Verification items for the finished model (mm, model axes). Round coordinates to 2 decimals unless told otherwise and drop trailing zeros. Loops run counter-clockwise (first coordinate to the right, second up) from the corner with the lowest first, then second, coordinate; pieces in that order, holes last. Notation, with made-up numbers: (77.25, -26.75) -> (136.25, -26.75) arc R20 cw to (136.25, 2.25) -> close; hole circle Ø2 at (-3.5, 19.5). An arc over 180 degrees is marked (long way). Use a Markdown table: item, result. Add a question column.
```python
from build123d import *

# Parameters (mm, degrees)
F0_R     = 44.45
F0_R_2   = 1.5
F0_R_3   = 2.5
F1_DEPTH = 3.175


# Not quite as in the source:
# - a length typed as a fraction of an inch, garbled in the dataset ("3 / 203.2 mm" for 3/8 in), is restored


with BuildPart() as f1:
    # F0 (on Front) → F1 (new body)
    with BuildSketch(Plane.XZ):
        Circle(F0_R)
        with Locations((-19.725, -34.1647021793)):
            Circle(F0_R_2, mode=Mode.SUBTRACT)
        with Locations((-34.1647021793, -19.725)):
            Circle(F0_R_2, mode=Mode.SUBTRACT)
        with Locations((0, -39.45)):
            Circle(F0_R_2, mode=Mode.SUBTRACT)
        with Locations((19.725, -34.1647021793)):
            Circle(F0_R_2, mode=Mode.SUBTRACT)
        Polygon((10, -27.5), (10, -15), (10, -2.5), (13.175, -2.5), (13.175, -15), (13.175, -27.5), align=None, mode=Mode.SUBTRACT)
        with Locations((34.1647021793, -19.725)):
            Circle(F0_R_2, mode=Mode.SUBTRACT)
        with Locations((-39.45, 0)):
            Circle(F0_R_2, mode=Mode.SUBTRACT)
        with Locations((-24.125, 9.91)):
            Circle(F0_R_3, mode=Mode.SUBTRACT)
        with Locations((-34.1647021793, 19.725)):
            Circle(F0_R_2, mode=Mode.SUBTRACT)
        with Locations((-24.125, 19.91)):
            Circle(F0_R_3, mode=Mode.SUBTRACT)
        with Locations((-19.725, 34.1647021793)):
            Circle(F0_R_2, mode=Mode.SUBTRACT)
        Polygon((-20, 15.91), (-20, 24.82), (20, 24.82), (20, 15.91), (30, 15.91), (30, 13.91), (20, 13.91), (20, 5), (-20, 5), (-20, 13.91), (-30, 13.91), (-30, 15.91), align=None, mode=Mode.SUBTRACT)
        with Locations((24.125, 9.91)):
            Circle(F0_R_3, mode=Mode.SUBTRACT)
        with Locations((39.45, 0)):
            Circle(F0_R_2, mode=Mode.SUBTRACT)
        with Locations((24.125, 19.91)):
            Circle(F0_R_3, mode=Mode.SUBTRACT)
        with Locations((34.1647021793, 19.725)):
            Circle(F0_R_2, mode=Mode.SUBTRACT)
        with Locations((0, 39.45)):
            Circle(F0_R_2, mode=Mode.SUBTRACT)
        with Locations((19.725, 34.1647021793)):
            Circle(F0_R_2, mode=Mode.SUBTRACT)
    extrude(amount=F1_DEPTH)


solid = f1.part
```
1) Sectioned sample at D-D on z = 9.91. Enter the section's corners in (x, y) (3 decimals), then the cut area to 3 significant figures.
2) Go/stop test with flat-tipped pins: pin 1 (1.6 mm diameter, centred on x = -24, y = -2, fed in from -Z); pin 2 (1.5 mm diameter, centred on x = 0, y = -0.5, fed in from +Z); pin 3 (1.6 mm diameter, centred on x = -24, y = -1.5, fed in from +Z); pin 4 (4.5 mm diameter, centred on x = 24.125, z = 9.91, fed in from +Y). Record where each tip stops, or that it passes through.
3) Sectioned sample at C-C on x = -39.45. Enter the section's corners in (y, z) (3 decimals).
4) Thickness scan on line 1 (Z direction, x = 0, y = -1.7); line 2 (X direction, y = -3, z = 21.5); line 3 (X direction, y = -0.5, z = 19.5). Record the ranges inside material, lowest first.
5) Sectioned sample at A-A on z = 0. Enter the section's corners in (x, y) (3 decimals).
6) Sectioned sample at B-B on y = -1.2. State how many separate pieces and enclosed holes the cut face has, then the cut area to 3 significant figures.
Geometry results:
| question | item | result |
|---|---|---|
| 1 | outline | (-43.331, -3.175) -> (-26.625, -3.175) -> (-26.625, 0) -> (-43.331, 0) -> close; (-21.625, -3.175) -> (-20, -3.175) -> (-20, 0) -> (-21.625, 0) -> close; (20, -3.175) -> (21.625, -3.175) -> (21.625, 0) -> (20, 0) -> close; (26.625, -3.175) -> (43.331, -3.175) -> (43.331, 0) -> (26.625, 0) -> close |
| 1 | area | 116 mm^2 |
| 2 | pin 1 | z = -37.92 |
| 2 | pin 2 | z = 44.45 |
| 2 | pin 3 | z = 37.92 |
| 2 | pin 4 | through |
| 3 | outline | (-3.175, -20.482) -> (0, -20.482) -> (0, -1.5) -> (-3.175, -1.5) -> close; (-3.175, 1.5) -> (0, 1.5) -> (0, 20.482) -> (-3.175, 20.482) -> close |
| 4 | line 1 | -44.45 to -40.95, -37.95 to 5, 24.82 to 37.95, 40.95 to 44.45 |
| 4 | line 2 | -38.9 to -26.05, -22.2 to -20, 20 to 22.2, 26.05 to 38.9 |
| 4 | line 3 | -39.94 to -35.65, -32.68 to -26.59, -21.66 to -20, 20 to 21.66, 26.59 to 32.68, 35.65 to 39.94 |
| 5 | outline | (-44.45, -3.175) -> (-40.95, -3.175) -> (-40.95, 0) -> (-44.45, 0) -> close; (-37.95, -3.175) -> (37.95, -3.175) -> (37.95, 0) -> (-37.95, 0) -> close; (40.95, -3.175) -> (44.45, -3.175) -> (44.45, 0) -> (40.95, 0) -> close |
| 6 | separate pieces | 1 |
| 6 | enclosed holes | 18 |
| 6 | area | 5,130 mm^2 |
